Can you work these out from the drawing? Everything is in mm from the part's minimum corner. A direction names the side the tool comes from. Give positions to 0.01 mm unless a question says otherwise; leave off trailing zeros. Write each loop counter-clockwise with the first axis right and the second up, starting at its lowest first coordinate (ties: lowest second). Pieces come first, ordered by that corner, then holes. Notation, with made-up numbers: (61.5, 10.5) - (108.5, 10.5) arc R16 cw to (108.5, 18.5) - close; hole circle Ø1 at (68.25, -39.75). An arc over 180 degrees is marked (long way). Answer in a Markdown table with one row per item.
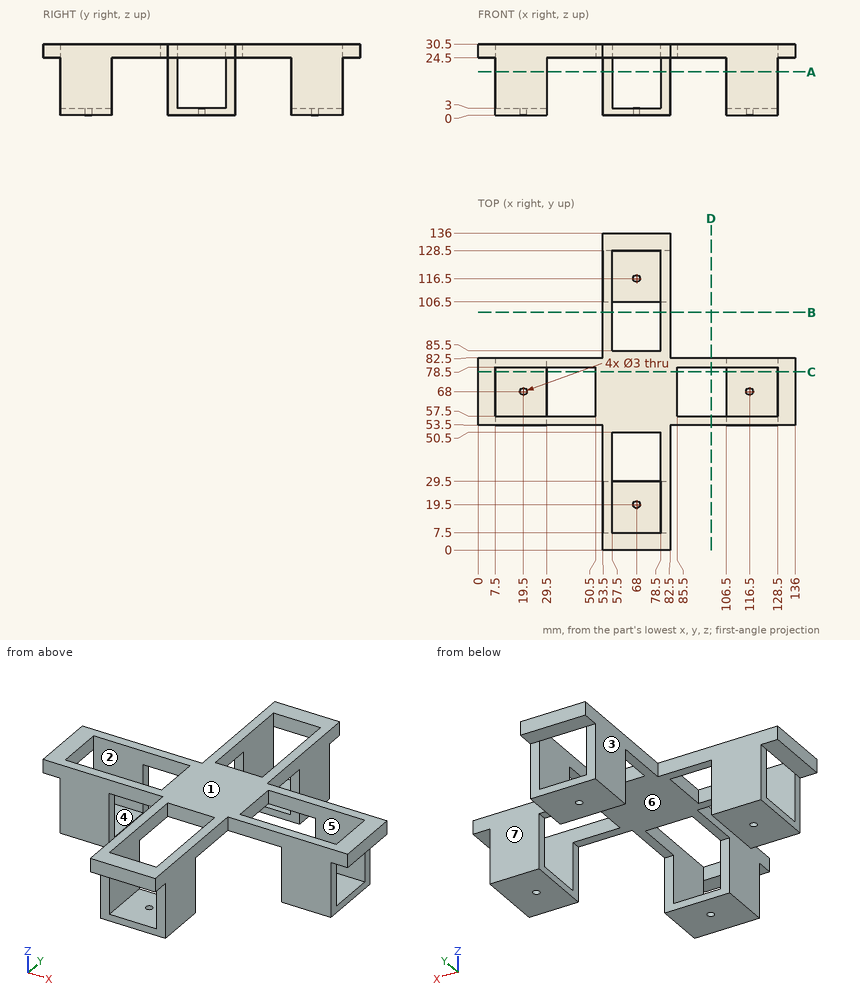
1) We'd pull the mould along X, two halves only. Please class the marked faces 1, 2 and 3: +X half, -X half, draft (parallel to the pull), parting line (faces both ways), or undercut.
Check values:
| item | result |
|---|---|
| face 1 | draft |
| face 2 | undercut |
| face 3 | -X half |
2) Will these pins go through, and if not, where does the flat tip stop? P1, Ø3.5, axis at x = 19.5, y = 68, coming from the +Z side; P2, Ø12, axis at y = 62.5, z = 12.5, coming from the +X side; P3, Ø14, axis at x = 107.5, z = 16.5, coming from the +Y side.
Check values:
| item | result |
|---|---|
| P1 | stops at z = 3 |
| P2 | stops at x = 128.5 |
| P3 | stops at y = 82.5 |
3) If I drill on line 1 (X direction, y = 68, z = 1); line 2 (Y direction, x = 101.5, z = 25), over which ranges is the centre line in solid material (lowest first)?
Check values:
| item | result |
|---|---|
| line 1 | x = 7.5 to 18, 21 to 29.5, 106.5 to 115, 118 to 128.5 |
| line 2 | y = 53.5 to 57.5, 78.5 to 82.5 |
4) Imagine slicing it at B-B (y = 102). List the corners of the cut face in (x, z) for me.
Check values:
| item | result |
|---|---|
| outline | (53.5, 24.5) - (57.5, 24.5) - (57.5, 30.5) - (53.5, 30.5) - close; (78.5, 24.5) - (82.5, 24.5) - (82.5, 30.5) - (78.5, 30.5) - close |
5) On a 3-axis mill with a long thin cutter (end or side, diameter ignored), from which of +Z, -Z, +X, -X, +Y, -Y can I reach the whole of each face in a straight line? I mean the marked faces 4, 5, 6 and 7. Say none if no direction works.
Check values:
| item | result |
|---|---|
| face 4 | +Z, +X, -X |
| face 5 | +Z |
| face 6 | -Z |
| face 7 | +Z, -Z, +X, +Y |
6) Imagine slicing it at A-A (z = 18.5). State how many separate pieces and enclosed holes the cut face has, then the cut area to 3 significant figures.
Check values:
| item | result |
|---|---|
| separate pieces | 8 |
| enclosed holes | 0 |
| area | 704 mm2 |
7) Imagine slicing it at C-C (y = 76.5). List the corners of the cut face in (x, z) for me, then the cut area to 3 significant figures.
Check values:
| item | result |
|---|---|
| outline | (0, 24.5) - (7.5, 24.5) - (7.5, 30.5) - (0, 30.5) - close; (7.5, 0) - (29.5, 0) - (29.5, 3) - (7.5, 3) - close; (50.5, 24.5) - (85.5, 24.5) - (85.5, 30.5) - (50.5, 30.5) - close; (106.5, 0) - (128.5, 0) - (128.5, 3) - (106.5, 3) - close; (128.5, 24.5) - (136, 24.5) - (136, 30.5) - (128.5, 30.5) - close |
| area | 432 mm2 |
